from build123d import *

# Parameters (mm, degrees)
F1_DEPTH  = 5
F3_DEPTH  = 25
F5_DEPTH  = 25
F6_R      = 2.5
F7_DEPTH  = 25
F8_R      = 2.5
F9_DEPTH  = 25
F10_W     = 20
F10_H     = 30
F11_DEPTH = 2
F13_R     = 2.5
F14_DEPTH = 10


with BuildPart() as f1:
    # F0 (on Front) → F1 (new body, symmetric)
    with BuildSketch(Plane.XZ):
        Polygon((0, 50), (0, 0), (2, 0), (2, 10), (2, 40), (2, 50), align=None)
    extrude(amount=F1_DEPTH, both=True)


with BuildPart() as f1b:
    # F0 (on Front) → F1, piece 2 (new body, symmetric)
    with BuildSketch(Plane.XZ):
        Polygon((22, 40), (22, 10), (22, 0), (24, 0), (24, 50), (22, 50), align=None)
    extrude(amount=F1_DEPTH, both=True)


with BuildPart() as f3_tool:
    # F2 (on face) → F3 (new body)
    with BuildSketch(Plane(origin=(0, 0, 0), x_dir=(0, -1, 0), z_dir=(-1, 0, 0))):
        with BuildLine():
            ThreePointArc((5, 5), (3.5355339059, 1.4644660941), (0, 0))
            Line((0, 0), (5, 0))
            Line((5, 0), (5, 5))
        make_face()
        with BuildLine():
            ThreePointArc((0, 0), (-3.5355339059, 1.4644660941), (-5, 5))
            Line((-5, 5), (-5, 0))
            Line((-5, 0), (0, 0))
        make_face()
    extrude(amount=-F3_DEPTH)


with BuildPart() as f1_1:
    add(f1.part)

    # F3: cut by f3_tool
    add(f3_tool.part, mode=Mode.SUBTRACT)


with BuildPart() as f1b_1:
    add(f1b.part)

    # F3: cut by f3_tool
    add(f3_tool.part, mode=Mode.SUBTRACT)


with BuildPart() as f5_tool:
    # F4 (on face) → F5 (new body)
    with BuildSketch(Plane(origin=(0, 0, 0), x_dir=(0, -1, 0), z_dir=(-1, 0, 0))):
        with BuildLine():
            ThreePointArc((-5, 45), (-3.5355339059, 48.5355339059), (0, 50))
            Line((0, 50), (-5, 50))
            Line((-5, 50), (-5, 45))
        make_face()
        with BuildLine():
            ThreePointArc((0, 50), (3.5355339059, 48.5355339059), (5, 45))
            Line((5, 45), (5, 50))
            Line((5, 50), (0, 50))
        make_face()
    extrude(amount=-F5_DEPTH)


with BuildPart() as f1_2:
    add(f1_1.part)

    # F5: cut by f5_tool
    add(f5_tool.part, mode=Mode.SUBTRACT)


with BuildPart() as f1b_2:
    add(f1b_1.part)

    # F5: cut by f5_tool
    add(f5_tool.part, mode=Mode.SUBTRACT)


with BuildPart() as f7_tool:
    # F6 (on face) → F7 (new body)
    with BuildSketch(Plane(origin=(0, 0, 0), x_dir=(0, -1, 0), z_dir=(-1, 0, 0))):
        with Locations((0, 45)):
            Circle(F6_R)
    extrude(amount=-F7_DEPTH)


with BuildPart() as f1_3:
    add(f1_2.part)

    # F7: cut by f7_tool
    add(f7_tool.part, mode=Mode.SUBTRACT)


with BuildPart() as f1b_3:
    add(f1b_2.part)

    # F7: cut by f7_tool
    add(f7_tool.part, mode=Mode.SUBTRACT)


with BuildPart() as f9_tool:
    # F8 (on face) → F9 (new body)
    with BuildSketch(Plane(origin=(0, 0, 0), x_dir=(0, -1, 0), z_dir=(-1, 0, 0))):
        with Locations((0, 5)):
            Circle(F8_R)
    extrude(amount=-F9_DEPTH)


with BuildPart() as f1_4:
    add(f1_3.part)

    # F9: cut by f9_tool
    add(f9_tool.part, mode=Mode.SUBTRACT)


with BuildPart() as f1b_4:
    add(f1b_3.part)

    # F9: cut by f9_tool
    add(f9_tool.part, mode=Mode.SUBTRACT)


with BuildPart() as f11:
    # F10 (on face) → F11 (new body)
    with BuildSketch(Plane.XZ.offset(5)):
        with Locations((12, 25)):
            Rectangle(F10_W, F10_H)
    extrude(amount=-F11_DEPTH)


with BuildPart() as f1_5:
    add(f1_4.part)

    # F12: union F1b, F11
    add(f1b_4.part)
    add(f11.part)

    # F13 (on face) → F14 (cut)
    with BuildSketch(Plane.YZ.offset(24)):
        with BuildLine():
            ThreePointArc((-5, 45), (-3.5355339059, 48.5355339059), (0, 50))
            Line((0, 50), (-5, 50))
            Line((-5, 50), (-5, 45))
        make_face()
        with BuildLine():
            ThreePointArc((0, 50), (3.5355339059, 48.5355339059), (5, 45))
            Line((5, 45), (5, 50))
            Line((5, 50), (0, 50))
        make_face()
        with Locations((0, 45)):
            Circle(F13_R)
        with BuildLine():
            ThreePointArc((5, 5), (3.5355339059, 1.4644660941), (0, 0))
            Line((0, 0), (5, 0))
            Line((5, 0), (5, 5))
        make_face()
        with BuildLine():
            ThreePointArc((0, 0), (-3.5355339059, 1.4644660941), (-5, 5))
            Line((-5, 5), (-5, 0))
            Line((-5, 0), (0, 0))
        make_face()
        with Locations((0, 5)):
            Circle(F13_R)
    extrude(amount=-F14_DEPTH, mode=Mode.SUBTRACT)


solid = f1_5.part
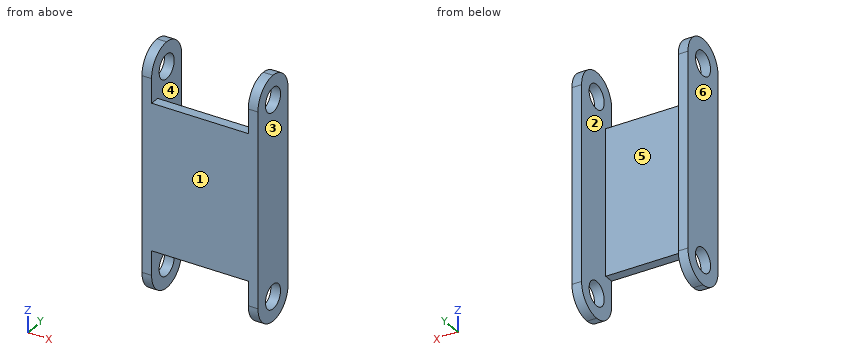
Check sheet for the modelled part. Datum: model origin and axes. Units: mm. Face numbers are marked on the shaded views. A direction names the side the tool comes from. Round coordinates to 2 decimals unless told otherwise and drop trailing zeros. Order: outer loops, then holes, each group sorted by start corner. A loop starts at its lowest first (then second) coordinate and runs counter-clockwise, first axis right, second up. Notation, with made-up numbers: M -34,86.5 L 6,86.5 A21 cw 6,92.5 Z; hole C 61.5,37 d6. An arc over 180 degrees is marked long. One line per item, written item: value. Start each with the question number.
1. Gauge pin test, flat ends, axial feed: P1, Ø0.6, axis at x = 7.5, y = -4, coming from the -Z side; P2, Ø4, axis at x = 13.5, y = -3, coming from the +Z side. Record the tip position at first contact, or that the pin passes through.
2. Section check A-A on y = 1.75. Enter the section's corners in (x, z), and give its area (3 significant figures).
3. Section check D-D on y = -3.5. Enter the section's corners in (x, z), and give its area (3 significant figures).
4. Release check for a two-part mould opening along X. For the marked faces 1, 2, 3 and 4 record: released by +X, released by -X, zero draft, split by the parting line, or undercut.
5. Access from +Z, -Z, +X, -X, +Y, -Y to the whole of each face (thin tool, end or side, straight path). Record for the marked faces 5 and 6.
6. Section check B-B on z = 34. Enter the section's corners in (x, y).
7. Scan lines: line 1 along Z through (x, y) = (23.2, 0); line 2 along X through (y, z) = (-1.75, 33); line 3 along Y through (x, z) = (22.55, 5). Record each from-to range of solid material in increasing order.
8. Section check C-C on x = 10.5. Enter the section's corners in (y, z).
Results found:
1. P1: z = 10
1. P2: z = 40
2. outline: M 0,0.32 L 2,0.32 L 2,3.21 L 0,3.21 Z; M 0,6.79 L 2,6.79 L 2,43.21 L 0,43.21 Z; M 0,46.79 L 2,46.79 L 2,49.68 L 0,49.68 Z; M 22,0.32 L 24,0.32 L 24,3.21 L 22,3.21 Z; M 22,6.79 L 24,6.79 L 24,43.21 L 22,43.21 Z; M 22,46.79 L 24,46.79 L 24,49.68 L 22,49.68 Z
2. area: 169 mm^2
3. outline: M 0,1.43 L 2,1.43 L 2,10 L 22,10 L 22,1.43 L 24,1.43 L 24,48.57 L 22,48.57 L 22,40 L 2,40 L 2,48.57 L 0,48.57 Z
3. area: 789 mm^2
4. face 1: zero draft
4. face 2: undercut
4. face 3: released by +X
4. face 4: undercut
5. face 5: +Z, -Z, +Y
5. face 6: +Z, -Z, -X, +Y, -Y
6. outline: M 0,-5 L 24,-5 L 24,5 L 22,5 L 22,-3 L 2,-3 L 2,5 L 0,5 Z
7. line 1: 0 to 2.5, 7.5 to 42.5, 47.5 to 50
7. line 2: 0 to 2, 22 to 24
7. line 3: -5 to -2.5, 2.5 to 5
8. outline: M -5,10 L -3,10 L -3,40 L -5,40 Z
